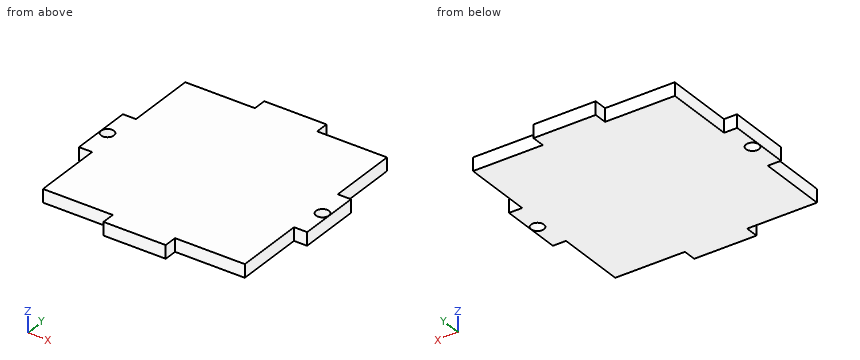
```python
from build123d import *

# Parameters (mm, degrees)
F1_W     = 48.65
F1_H     = 48.65
F2_DEPTH = 3.175
F3_W     = 3.175
F3_H     = 15
F3_W_2   = 15
F3_H_2   = 3.175
F4_DEPTH = 3.175
F5_R     = 1.55
F6_DEPTH = 3.176


with BuildPart() as f2:
    # F1 (on Top) → F2 (new body)
    with BuildSketch(Plane.XY):
        Rectangle(F1_W, F1_H)
    extrude(amount=F2_DEPTH)

    # F3 (on face) → F4 (join, through all)
    with BuildSketch(Plane.XY.offset(3.175)):
        with Locations((-25.9125, 0)):
            Rectangle(F3_W, F3_H)
        with Locations((0, 25.9125)):
            Rectangle(F3_W_2, F3_H_2)
        with Locations((0, -25.9125)):
            Rectangle(F3_W_2, F3_H_2)
        with Locations((25.9125, 0)):
            Rectangle(F3_W, F3_H)
    extrude(amount=-F4_DEPTH)

    # F5 (on face) → F6 (cut, through all)
    with BuildSketch(Plane.XY.offset(3.175)):
        with Locations((-25.9125, 0)):
            Circle(F5_R)
        with Locations((25.9125, 0)):
            Circle(F5_R)
    extrude(amount=-F6_DEPTH, mode=Mode.SUBTRACT)


solid = f2.part
```
Geometry check sheet. Reference: the model listing, model coordinates, mm. Coordinates: 2 decimals unless noted, no trailing zeros. Order: outer loops, then holes, each group sorted by start corner. A loop starts at its lowest first (then second) coordinate and runs counter-clockwise, first axis right, second up. Notation, with made-up numbers: (-19, -34) - (13, -34) arc R19 cw to (13, -11) - close; hole circle Ø6 at (23, 27.5). An arc over 180 degrees is marked (long way). Answer as a JSON object with one key per item and string values. Group by question number.
Item 1: Scan line: probe 1 along X at (y, z) = (-22, 2.85) (3 decimals). Record every from-to range of solid material in increasing order.
Item 2: Sectioned sample at A-A, the plane y = 0. Give the number of separate pieces and of enclosed holes in the cut face, and give its area (3 significant figures).
Item 3: Depth check by flat-ended pin: pin 1 Ø1 at (y, z) = (26.5, 2) entering from -X; pin 2 Ø1.5 at (x, z) = (20, 1.5) entering from +Y (3 decimals); pin 3 Ø1 at (x, z) = (19.5, 1) entering from -Y (3 decimals). Enter the tip coordinate at first touch or a pass-through.
Item 4: Sectioned sample at C-C, the plane x = 13. Record the cut outline in (y, z) (3 decimals).
Resolved:
{
 "1": {"probe 1": "-24.325 to 24.325"},
 "2": {"separate pieces": "3", "enclosed holes": "0", "area": "155 mm^2"},
 "3": {"pin 1": "x = -7.5", "pin 2": "y = 24.325", "pin 3": "y = -24.325"},
 "4": {"outline": "(-24.325, 0) - (24.325, 0) - (24.325, 3.175) - (-24.325, 3.175) - close"}
}
